Part print with two shaded views. Sizes in mm from the minimum x, y, z corner. Give positions to 0.01 mm unless a question says otherwise; leave off trailing zeros. Loops run counter-clockwise (first coordinate to the right, second up) from the corner with the lowest first, then second, coordinate; pieces in that order, holes last. Notation, with made-up numbers: (-11.5, 37.5) -> (32.5, 37.5) arc R14 cw to (32.5, 57.5) -> close; hole circle Ø2 at (1.25, 53.25). An arc over 180 degrees is marked (long way). One line per question, with ' | ' between items.
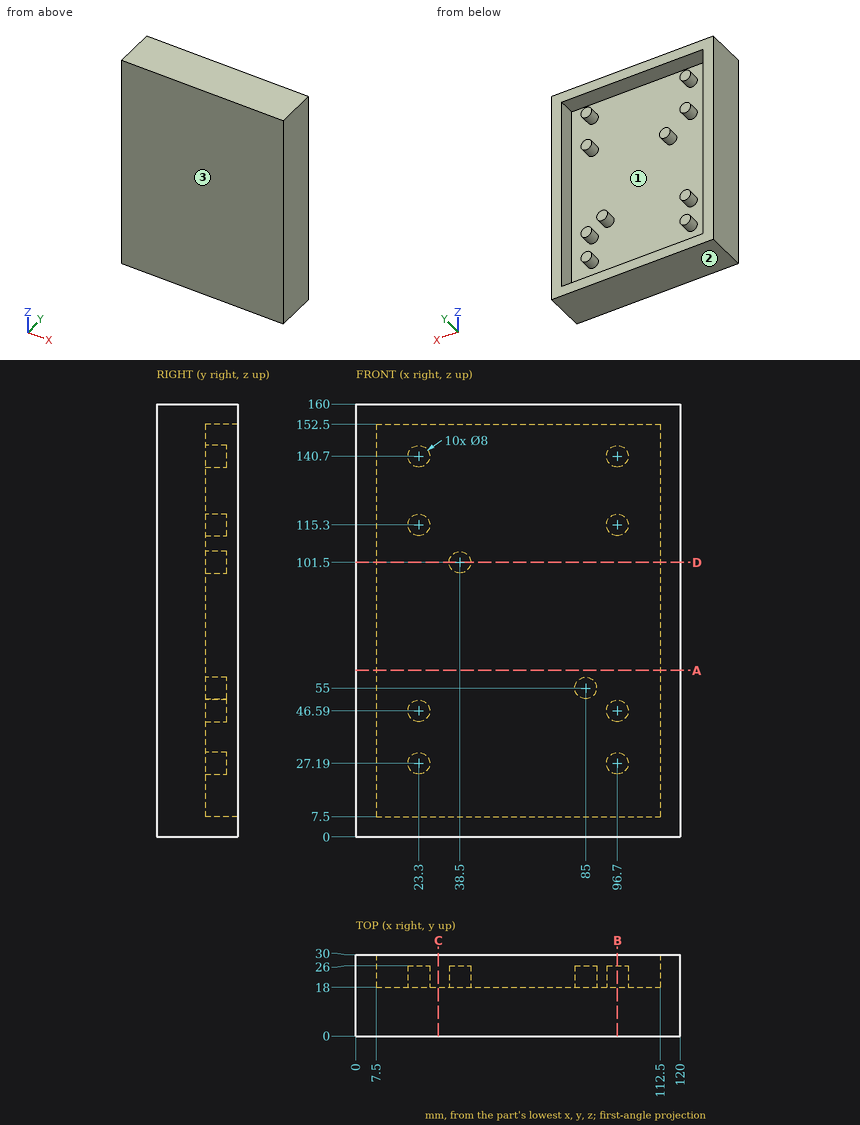
1) Drill centre lines: line 1 (Z direction, x = 104, y = 26.5); line 2 (X direction, y = 21.5, z = 104); line 3 (X direction, y = 24, z = 102.5). Where is each one in solid material? Low to high.
Found:
line 1: 0 to 7.5, 152.5 to 160 | line 2: 0 to 7.5, 35.38 to 41.62, 112.5 to 120 | line 3: 0 to 7.5, 34.63 to 42.37, 112.5 to 120
2) Saw through at A-A (z = 61.5). Give the cut face in (x, y), and give its area (3 significant figures).
Found:
outline: (0, 0) -> (120, 0) -> (120, 30) -> (112.5, 30) -> (112.5, 18) -> (7.5, 18) -> (7.5, 30) -> (0, 30) -> close | area: 2,340 mm2
3) Saw through at C-C (x = 30.5). Give the cut face in (y, z).
Found:
outline: (0, 0) -> (30, 0) -> (30, 7.5) -> (18, 7.5) -> (18, 152.5) -> (30, 152.5) -> (30, 160) -> (0, 160) -> close
4) Pull direction Z, two halves, no side cores. Call the marked faces 1, 2 and 3: pulls with the +Z half, pulls with the -Z half, needs draft (parallel to the pull), parting line crosses it, or undercut.
Found:
face 1: undercut | face 2: pulls with the -Z half | face 3: needs draft
5) Pin check, flat tips, straight feed: P1, Ø4, axis at x = 25, z = 48.5, coming from the +Y side; P2, Ø2, axis at x = 15, z = 70, coming from the +Y side. Stop position of each tip, or through.
Found:
P1: y = 26 | P2: y = 18
6) Saw through at D-D (z = 101.5). Give the cut face in (x, y).
Found:
outline: (0, 0) -> (120, 0) -> (120, 30) -> (112.5, 30) -> (112.5, 18) -> (42.5, 18) -> (42.5, 26) -> (34.5, 26) -> (34.5, 18) -> (7.5, 18) -> (7.5, 30) -> (0, 30) -> close
7) Saw through at B-B (x = 96.7). Give the cut face in (y, z), and give its area (3 significant figures).
Found:
outline: (0, 0) -> (30, 0) -> (30, 7.5) -> (18, 7.5) -> (18, 23.19) -> (26, 23.19) -> (26, 31.19) -> (18, 31.19) -> (18, 42.59) -> (26, 42.59) -> (26, 50.59) -> (18, 50.59) -> (18, 111.3) -> (26, 111.3) -> (26, 119.3) -> (18, 119.3) -> (18, 136.7) -> (26, 136.7) -> (26, 144.7) -> (18, 144.7) -> (18, 152.5) -> (30, 152.5) -> (30, 160) -> (0, 160) -> close | area: 3,320 mm2
